from build123d import *

# Parameters (mm, degrees)
EXTRUDE_1_DEPTH     = 18
SKETCH_2_R          = 1.15
CUT_EXTRUDE_1_DEPTH = 16
FILLET_1_R          = 3


with BuildPart() as part:
    # 草图1 → 凸台-拉伸1 (new body)
    with BuildSketch(Plane.XY):
        with BuildLine():
            Line((6, 0), (0, 0))
            Line((0, 0), (0, 12))
            Line((0, 12), (4, 12))
            ThreePointArc((4, 12), (5.414213562, 11.414213562), (6, 10))
            Line((6, 10), (6, 0))
        make_face()
    extrude(amount=EXTRUDE_1_DEPTH)

    # 草图2 → 切除-拉伸1 (cut)
    with BuildSketch(Plane.XZ):
        with Locations((3, 13.5)):
            Circle(SKETCH_2_R)
        with Locations((3, 4.5)):
            Circle(SKETCH_2_R)
    extrude(amount=-CUT_EXTRUDE_1_DEPTH, mode=Mode.SUBTRACT)

    # 圆角1
    fillet_1_edges = [part.edges().sort_by_distance(p)[0] for p in [
        (0, 6, 18),
        (0, 6, 0),
    ]]
    fillet(fillet_1_edges, radius=FILLET_1_R)


solid = part.part
For this review, take the finished solid that the model builds, in its own axes (mm). Round coordinates to 2 decimals unless told otherwise and drop trailing zeros. Order: outer loops, then holes, each group sorted by start corner. A loop starts at its lowest first (then second) coordinate and runs counter-clockwise, first axis right, second up. Notation, with made-up numbers: (6, 13) -> (40, 13) arc R22 ccw to (40, 52) -> close; hole circle Ø4 at (62, 60). An arc over 180 degrees is marked (long way). Put each result on its own line as item: value.
Q1. Add section D-D on z = 13.25. Write out the cut boundary in (x, y).
Check result:
outline: (0, 0) -> (1.88, 0) -> (1.88, 12) -> (0, 12) -> close; (4.12, 0) -> (6, 0) -> (6, 10) arc R2 ccw to (4.12, 12) -> close
Q2. Add section A-A on y = 7. Write out the cut boundary in (x, z).
Check result:
outline: (0, 3) arc R3 ccw to (3, 0) -> (6, 0) -> (6, 18) -> (3, 18) arc R3 ccw to (0, 15) -> close; hole circle Ø2.3 at (3, 4.5); hole circle Ø2.3 at (3, 13.5)
Q3. Add section C-C on z = 4.5. Write out the cut boundary in (x, y), plus the area to 3 significant figures.
Check result:
outline: (0, 0) -> (1.85, 0) -> (1.85, 12) -> (0, 12) -> close; (4.15, 0) -> (6, 0) -> (6, 10) arc R2 ccw to (4.15, 11.99) -> close
area: 43.5 mm2
Q4. For probe 1 along Z at (x, y) = (3, 7); probe 2 along X at (y, z) = (4.25, 4.5); probe 3 along Z at (x, y) = (2.5, 6.25), list the stretches that pass through material, from the lowest coordinate up. Write a range as [from, to].
Check result:
probe 1: [0, 3.35], [5.65, 12.35], [14.65, 18]
probe 2: [0, 1.85], [4.15, 6]
probe 3: [0.04, 3.46], [5.54, 12.46], [14.54, 17.96]
Q5. Add section B-B on x = 2.5. Write out the cut boundary in (y, z), plus the area to 3 significant figures.
Check result:
outline: (0, 0.04) -> (12, 0.04) -> (12, 3.46) -> (0, 3.46) -> close; (0, 5.54) -> (12, 5.54) -> (12, 12.46) -> (0, 12.46) -> close; (0, 14.54) -> (12, 14.54) -> (12, 17.96) -> (0, 17.96) -> close
area: 165 mm2
Q6. Mouldability with a two-part tool opening along X and no side actions: class faces 1 (the flat face through (5, 6, 0)), 2 (the cylindrical face through (5.4, 11.43, 8.87)), 3 (the cylindrical face through (2.85, 5.92, 5.64)), 4 (the cylindrical face through (2.09, 5.92, 12.8)) as pulls with the +X half, pulls with the -X half, needs draft (parallel to the pull), parting line crosses it, or undercut.
Check result:
face 1: needs draft
face 2: pulls with the +X half
face 3: undercut
face 4: undercut
